Work out the finished part from the listing and answer in its coordinate system (mm). A direction names the side the tool comes from. Coordinates: 2 decimals unless noted, no trailing zeros. Order: outer loops, then holes, each group sorted by start corner. A loop starts at its lowest first (then second) coordinate and runs counter-clockwise, first axis right, second up. Notation, with made-up numbers: M 33,40.25 L 85,40.25 A35 ccw 85,74.25 Z; hole C -20,1 d9. An arc over 180 degrees is marked long. Use a Markdown table: item, result.
Autodesk Inventor part; units mm, degrees
ref_plane "YZ Plane" through (0, 0, 0) normal (1, 0, 0) x (0, 1, 0)
ref_plane "XZ Plane" through (0, 0, 0) normal (0, 1, 0) x (-1, 0, 0)
ref_plane "XY Plane" through (0, 0, 0) normal (0, 0, 1) x (1, 0, 0)
sketch "Esquisse1" plane through (0, 0, 0) normal (0, 0, 1) x (1, 0, 0)
  line L0 (0, 0) -> (41, 0)
  line L1 (41, 0) -> (41, 38)
  line L2 (41, 38) -> (0, 38)
  line L3 (0, 38) -> (0, 0)
  dimension "d0" = 41
  dimension "d1" = 38
extrude "Extrusion1" add sketch "Esquisse1" along normal blind 20
sketch "Esquisse2" plane through (0, 38, 0) normal (0, 1, 0) x (1, 0, 0)
  line L0 (0, 0) -> (0, -20)
  line L1 (0, -10) -> (0, -15)
  line L2 (0, -15) -> (0, -6.5)
  line L3 (0, -10) -> (38, -10)
  line L4 (38, -10) -> (38, -2.5)
  line L5 (38, -2.5) -> (4, -2.5)
  line L6 (0, -2.5) -> (0, -10)
  line L7 (38, -10) -> (38, -17.5)
  line L8 (38, -17.5) -> (4, -17.5)
  line L9 (0, -13.5) -> (0, -10)
  arc A0 (0, -13.5) -> (4, -17.5) centre (4, -13.5) ccw
  arc A1 (4, -2.5) -> (0, -6.5) centre (4, -6.5) ccw
  point P0 (0, -5)
  point P1 (0, -17.5)
  point P2 (0, -2.5)
  point P3 (0, -17.5)
  point P4 (0, -13.5)
  dimension "d6" = 38
  dimension "d9" = 15
  dimension "d10" = 4
  dimension "d11" = 4
extrude "Extrusion2" add sketch "Esquisse2" along normal blind 2
sketch "Esquisse3" plane through (0, 40, 0) normal (0, 1, 0) x (1, 0, 0)
  line L0 (4, -17.5) -> (38, -17.5)
  line L1 (0, -6.5) -> (0, -13.5)
  line L2 (2.9996, -7) -> (8.9996, -7)
  line L3 (8.9996, -7) -> (8.9996, -13)
  line L4 (8.9996, -13) -> (2.9996, -13)
  line L5 (2.9996, -13) -> (2.9996, -7)
  line L6 (2.9996, -7) -> (8.9996, -13) construction
  line L7 (8.9996, -7) -> (2.9996, -13) construction
  point P0 (0, 0)
  point P1 (5.9996, -10)
  dimension "d12" = 7.5
  dimension "d13" = 5.9996
  dimension "d14" = 6
  dimension "d15" = 6
extrude "Extrusion3" add sketch "Esquisse3" along normal blind 10
sketch "Esquisse4" plane through (8.9996, 40, 7) normal (0, 0, -1) x (-1, 0, 0)
  line L0 (6, 10) -> (0, 10)
  line L1 (0, 10) -> (6, 10)
  line L2 (6, 10) -> (6, 7.5)
  line L3 (6, 7.5) -> (0, 7.5)
  line L4 (0, 7.5) -> (0, 10)
  point P0 (8.9996, -40)
  dimension "d18" = 6
  dimension "d19" = 2.5
extrude "Extrusion4" add sketch "Esquisse4" along normal blind 15
sketch "Esquisse6" plane through (2.9996, 40, 13) normal (0, 0, 1) x (1, 0, 0)
  line L0 (0, 10) -> (6, 10)
  line L1 (0, 10) -> (6, 10)
  line L2 (6, 10) -> (6, 7.5)
  line L3 (6, 7.5) -> (0, 7.5)
  line L4 (0, 7.5) -> (0, 10)
  point P0 (-2.9996, -40)
  dimension "d22" = 6
  dimension "d23" = 2.5
extrude "Extrusion5" add sketch "Esquisse6" along normal blind 15
fillet "Congé1" radius 3 4 edges at (2.9996, 43.75, 7) (2.9996, 43.75, 13) (8.9996, 43.75, 13) (8.9996, 43.75, 7)
sketch "Esquisse9" plane through (41, 0, 0) normal (1, 0, 0) x (0, 0, -1)
  line L0 (-20, 0) -> (-20, 38)
  line L1 (-20, 38) -> (-20, 31)
  line L2 (-20, 31) -> (-11, 31)
  line L3 (-11, 31) -> (-11, 28)
  line L4 (-11, 28) -> (-20, 28)
  line L5 (-20, 28) -> (-20, 31)
  line L6 (-11, 31) -> (-10, 31)
  line L7 (0, 31) -> (-9, 31)
  line L8 (-9, 31) -> (-9, 28)
  line L9 (-9, 28) -> (0, 28)
  line L10 (0, 28) -> (0, 31)
  point P0 (0, 0)
  dimension "d38" = 7
  dimension "d39" = 9
  dimension "d40" = 3
  dimension "d41" = 1
extrude "Extrusion9" add sketch "Esquisse9" along normal blind 5
sketch "Esquisse10" plane through (0, 0, 0) normal (-1, 0, 0) x (0, 0, 1)
  line L0 (0, 38) -> (0, 31)
  line L1 (0, 38) -> (0, 0)
  line L2 (0, 31) -> (9, 31)
  line L3 (9, 31) -> (9, 28)
  line L4 (9, 28) -> (0, 28)
  line L5 (0, 28) -> (0, 31)
  line L6 (9, 31) -> (10, 31)
  line L7 (10, 31) -> (10, 24.8436)
  line L8 (20, 31) -> (11, 31)
  line L9 (11, 31) -> (11, 28)
  line L10 (11, 28) -> (20, 28)
  line L11 (20, 28) -> (20, 31)
  dimension "d44" = 7
  dimension "d45" = 9
  dimension "d46" = 3
  dimension "d47" = 1
extrude "Extrusion10" add sketch "Esquisse10" along normal blind 5
properties part number "Servomoteur analogique FS5106B"
(1) Determine the mould class of faces 5 (the flat face through (6, 47.5, -1)), 6 (the flat face through (41, 19, 10)), 7 (the flat face through (-2, 28, 15)) for opening direction Y: pulls with the +Y half, pulls with the -Y half, needs draft (parallel to the pull), parting line crosses it, or undercut.
Conclusion:
| item | result |
|---|---|
| face 5 | undercut |
| face 6 | needs draft |
| face 7 | pulls with the -Y half |
(2) A cutting plane is placed at A-A (x = 42). Determine the outline of the cut face in (y, z), then the cut area to 3 significant figures.
Conclusion:
| item | result |
|---|---|
| outline | M 28,0 L 31,0 L 31,9 L 28,9 Z; M 28,11 L 31,11 L 31,20 L 28,20 Z |
| area | 54.0 mm2 |
(3) A cutting plane is placed at D-D (x = 21). Determine the outline of the cut face in (y, z).
Conclusion:
| item | result |
|---|---|
| outline | M 0,0 L 38,0 L 38,2.5 L 40,2.5 L 40,17.5 L 38,17.5 L 38,20 L 0,20 Z |
(4) Given P1, Ø4, axis at x = 8, y = 33, coming from the +Z side; P2, Ø2.5, axis at x = -3, y = 29, coming from the -Z side; P3, Ø0.6, axis at x = 20.5, y = 38.5, coming from the +Z side, each flat-ended and moving along its own axis, determine where each tip first touches the part or whether it passes through.
Conclusion:
| item | result |
|---|---|
| P1 | z = 20 |
| P2 | z = 0 |
| P3 | z = 17.5 |
(5) A cutting plane is placed at C-C (z = 4). Determine the outline of the cut face in (x, y), then the cut area to 3 significant figures.
Conclusion:
| item | result |
|---|---|
| outline | M -5,28 L 0,28 L 0,0 L 41,0 L 41,28 L 46,28 L 46,31 L 41,31 L 41,38 L 38,38 L 38,40 L 0.88,40 L 0.88,38 L 0,38 L 0,31 L -5,31 Z; M 3,47.5 L 9,47.5 L 9,50 L 3,50 Z |
| area | 1,680 mm2 |
(6) Straight lines are drawn through the part: L1, parallel to Y at x = 8, z = 19.5; L2, parallel to X at y = 13.5, z = 9.5; L3, parallel to Z at x = 38, y = 3.5. For each, find the intervals that lie inside material, in ascending order.
Conclusion:
| item | result |
|---|---|
| L1 | 0 to 38, 47.5 to 50 |
| L2 | 0 to 41 |
| L3 | 0 to 20 |
(7) Which of the six approach directions +Z, -Z, +X, -X, +Y, -Y give full straight-line access (tool end or side, diameter ignored) to faces 1 (the flat face through (43, 30, 11)), 2 (the flat face through (-2, 30, 9)), 3 (the flat face through (43, 31, 16)), 4 (the flat face through (20, 19, 20))?
Conclusion:
| item | result |
|---|---|
| face 1 | +X, +Y, -Y |
| face 2 | -X, +Y, -Y |
| face 3 | +Z, -Z, +X, +Y |
| face 4 | +Z, +X, -X, -Y |
